```python
from build123d import *

# Parameters (mm, degrees)
ESQUISSE1_W             = 22.16
ESQUISSE1_H             = 40
BOSS_EXTRU_1_DEPTH      = 40
CHANFREIN1_SIZE         = 11
CHANFREIN1_SIZE2        = 21
CHANFREIN2_SIZE         = 11
CHANFREIN2_SIZE2        = 21
CONG_1_R                = 4
ESQUISSE2_R             = 4
BOSS_EXTRU_2_DEPTH      = 40
ESQUISSE2_3_R           = 4
BOSS_EXTRU_3_DEPTH      = 40
ESQUISSE3_R             = 12.5
BOSS_EXTRU_4_DEPTH      = 6
ESQUISSE4_R             = 16
ENL_V_MAT_EXTRU_1_DEPTH = 7.2
ESQUISSE6_W             = 12.088624029
ESQUISSE6_H             = 7.650078289
ENL_V_MAT_EXTRU_2_DEPTH = 86.171439898
CONG_2_R                = 2
ESQUISSE8_R             = 5.5
ENL_V_MAT_EXTRU_5_DEPTH = 15


with BuildPart() as part:
    # Esquisse1 → Boss.-Extru.1 (new body)
    with BuildSketch(Plane(origin=(0, 0, 0), x_dir=(1, 0, 0), z_dir=(0, 1, 0))):
        with Locations((26.894106866, -0.367930046)):
            Rectangle(ESQUISSE1_W, ESQUISSE1_H)
    extrude(amount=BOSS_EXTRU_1_DEPTH)

    # Chanfrein1
    chanfrein1_edges = [part.edges().sort_by_distance(p)[0] for p in [
        (26.894106866, 0, 20.367930046),
    ]]
    chanfrein1_side = [part.faces().sort_by_distance(p)[0] for p in [
        (26.894106866, 0, 0.367930046),
    ]]
    chamfer(chanfrein1_edges, length=CHANFREIN1_SIZE, length2=CHANFREIN1_SIZE2, reference=chanfrein1_side[0])

    # Chanfrein2
    chanfrein2_edges = [part.edges().sort_by_distance(p)[0] for p in [
        (26.894106866, 0, -19.632069954),
    ]]
    chanfrein2_side = [part.faces().sort_by_distance(p)[0] for p in [
        (26.894106866, 0, -5.132069954),
    ]]
    chamfer(chanfrein2_edges, length=CHANFREIN2_SIZE, length2=CHANFREIN2_SIZE2, reference=chanfrein2_side[0])

    # Cong_1
    cong_1_edges = [part.edges().sort_by_distance(p)[0] for p in [
        (26.894106866, 0, 9.367930046),
    ]]
    fillet(cong_1_edges, radius=CONG_1_R)

    # Esquisse2 → Boss.-Extru.2 (add)
    with BuildSketch(Plane(origin=(0, 40, 0), x_dir=(1, 0, 0), z_dir=(0, 1, 0))):
        with Locations(Location((23.814106866, 11.632069954, 0), (0, 0, 270))):
            Circle(ESQUISSE2_R)
    extrude(amount=BOSS_EXTRU_2_DEPTH)

    # Esquisse2_3 → Boss.-Extru.3 (add)
    with BuildSketch(Plane(origin=(0, 40, 0), x_dir=(1, 0, 0), z_dir=(0, 1, 0))):
        with Locations(Location((23.814106866, -12.367930046, 0), (0, 0, 270))):
            Circle(ESQUISSE2_3_R)
        with Locations(Location((23.814106866, 11.632069954, 0), (0, 0, 270))):
            Circle(ESQUISSE2_3_R)
    extrude(amount=BOSS_EXTRU_3_DEPTH)

    # Esquisse3 → Boss.-Extru.4 (add)
    with BuildSketch(Plane.ZY.offset(-15.814106866)):
        with Locations(Location((0.367930046, 13.5, 0), (0, 0, 180))):
            Circle(ESQUISSE3_R)
    extrude(amount=BOSS_EXTRU_4_DEPTH)

    # Esquisse4 → Enl_v. mat.-Extru.1 (cut)
    with BuildSketch(Plane(origin=(37.974106866, 0, 0), x_dir=(0, 0, -1), z_dir=(1, 0, 0))):
        with Locations((-1.650800507, 12.8)):
            Circle(ESQUISSE4_R)
    extrude(amount=-ENL_V_MAT_EXTRU_1_DEPTH, mode=Mode.SUBTRACT)

    # Esquisse6 → Enl_v. mat.-Extru.2 (cut, through all)
    with BuildSketch(Plane(origin=(30.774106866, 0, 0), x_dir=(0, 0, -1), z_dir=(1, 0, 0))):
        with Locations((6.871590707, 0.920255373)):
            Rectangle(ESQUISSE6_W, ESQUISSE6_H)
    extrude(amount=ENL_V_MAT_EXTRU_2_DEPTH, mode=Mode.SUBTRACT)

    # Cong_2
    cong_2_edges = [part.edges().sort_by_distance(p)[0] for p in [
        (23.294106866, 0, -8.632069954),
    ]]
    fillet(cong_2_edges, radius=CONG_2_R)

    # Esquisse8 → Enl_v. mat.-Extru.5 (cut)
    with BuildSketch(Plane(origin=(37.974106866, 0, -37.974106866), x_dir=(0, 0, 1), z_dir=(-1, 0, 0))):
        with Locations(Location((38.342036913, 12.8, 0), (0, 0, 180))):
            Circle(ESQUISSE8_R)
    extrude(amount=ENL_V_MAT_EXTRU_5_DEPTH, mode=Mode.SUBTRACT)


solid = part.part
```
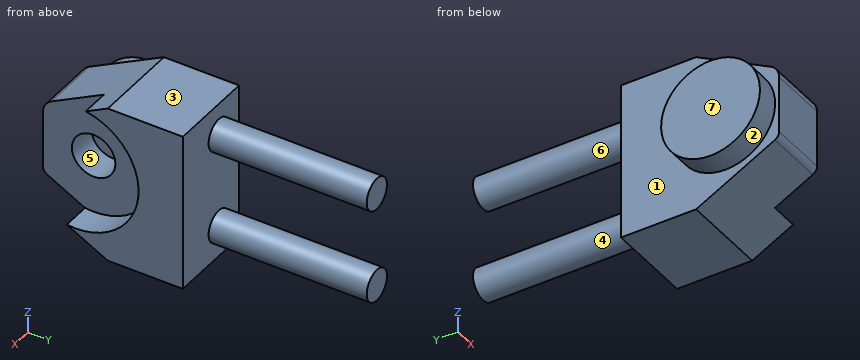
Could you check a few things on this model? Use its own coordinates, in mm. Face numbers are marked on the shaded views. A direction names the side the tool comes from. Coordinates: 2 decimals unless noted, no trailing zeros. Loops run counter-clockwise (first coordinate to the right, second up) from the corner with the lowest first, then second, coordinate; pieces in that order, holes last.
1) Imagine slicing it at C-C (z = 2). List the corners of the cut face in (x, y) for me.
Reported:
outline: (9.81, 1.11) - (15.81, 1.11) - (15.81, 0) - (30.77, 0) - (30.77, 7.55) - (22.97, 7.55) - (22.97, 18.05) - (30.77, 18.05) - (30.77, 28.8) - (37.97, 28.8) - (37.97, 40) - (15.81, 40) - (15.81, 25.89) - (9.81, 25.89) - close
2) Please list where these lines run through material, in increasing order: line 1 along X through (y, z) = (29, 0.5); line 2 along Z through (x, y) = (26.25, 12.8); line 3 along X through (y, z) = (16, -10.5).
Reported:
line 1: x = 15.81 to 37.97
line 2: z = -15.34 to -5.13, 5.87 to 16.07
line 3: x = 9.81 to 30.77
3) Imagine slicing it at D-D (z = 14). List the corners of the cut face in (x, y) for me.
Reported:
outline: (15.81, 8.84) - (30.77, 8.84) - (30.77, 22.97) - (37.97, 22.97) - (37.97, 40) - (27.47, 40) - (27.47, 80) - (20.16, 80) - (20.16, 40) - (15.81, 40) - close
4) Thinking about a two-plate mould opening in Z: for the marked faces 1, 2, 3 and 4, which applies, released by +Z, released by -Z, zero draft, split by the parting line, or undercut?
Reported:
face 1: zero draft
face 2: split by the parting line
face 3: released by +Z
face 4: undercut
5) Will these pins go through, and if not, where does the flat tip stop? pin 1 Ø1 at (x, y) = (24.5, 19.5) entering from -Z; pin 2 Ø5.5 at (y, z) = (10.5, -1) entering from +X; pin 3 Ø6 at (y, z) = (11.5, 14) entering from +X.
Reported:
pin 1: stops at z = -19.11
pin 2: stops at x = 22.97
pin 3: stops at x = 30.77
6) Which directions (+Z, -Z, +X, -X, +Y, -Y) give clear straight access to the entire face, cutting with the end or side of a thin tool? Please do the marked faces 5, 6 and 7.
Reported:
face 5: +X
face 6: +Y
face 7: +Z, -Z, -X, +Y, -Y
7) Imagine slicing it at B-B (y = 9). List the corners of the cut face in (x, z) for me.
Reported:
outline: (9.81, -11.29) - (15.81, -11.29) - (15.81, -13.35) - (30.77, -13.35) - (30.77, -3.61) - (22.97, -3.61) - (22.97, 4.34) - (30.77, 4.34) - (30.77, 14.08) - (15.81, 14.08) - (15.81, 12.03) - (9.81, 12.03) - close
8) Imagine slicing it at A-A (x = 17.5). List the corners of the cut face in (y, z) for me, and give its area (3 significant figures).
Reported:
outline: (0, -7.42) arc R2 ccw to (1.07, -9.19) - (21, -19.63) - (40, -19.63) - (40, 20.37) - (21, 20.37) - (2.14, 10.49) arc R4 ccw to (0, 6.95) - close
area: 1,370 mm2
